Work out the finished part from the listing and answer in its coordinate system (mm). A direction names the side the tool comes from. Give positions to 0.01 mm unless a question says otherwise; leave off trailing zeros. Loops run counter-clockwise (first coordinate to the right, second up) from the corner with the lowest first, then second, coordinate; pieces in that order, holes last. Notation, with made-up numbers: (32.25, 66) -> (87.25, 66) arc R12 cw to (87.25, 80) -> close; hole circle Ø7 at (38.25, 23.5). An arc over 180 degrees is marked (long way). Answer as CSV lines item,"result". Start each with the question number.
1. Determine the mould class of faces 1 (the face through (1, 21, 1.473)), 2 (the face through (28.02, 0.73, 9.95)), 3 (the face through (-33.65, 10.52, 0.75)) for opening direction Z: +Z half, -Z half, draft (parallel to the pull), parting line (faces both ways), or undercut.
2. Find the intervals of material crossed by line 1 along Y through (x, z) = (0.5, 17); line 2 along Z through (x, y) = (30, 1), in increasing order.
3. A tool of negligible diameter and unlimited length cuts with its end or side. For faces 4 (the face through (38.27, 30.52, 0.73)), 5 (the face through (1, 1.473, 21)), from which of +Z, -Z, +X, -X, +Y, -Y can it reach the whole face along a straight path? Write none if from no direction.
4. Flat-ended cylindrical pins translate along their axes: pin 1 Ø5 at (x, y) = (15.5, 13.5) entering from +Z; pin 2 Ø1.5 at (x, z) = (6.5, 9) entering from +Y. Find the tip coordinate at first contact, or state that the pin passes through.
5. Find section A-A, the plane x = 30. Give the vertices of the cut face in (y, z).
6. Find section B-B, the plane y = 18. Give the vertices of the cut face in (x, z), and give its area (3 significant figures).
from build123d import *

# Parameters (mm, degrees)
F1_DEPTH = 50.8
F2_R     = 2.5
F3_DEPTH = 12.7
F4_R     = 2.5
F5_DEPTH = 12.7


with BuildPart() as f1:
    # F0 (on Right) → F1 (new body, symmetric)
    with BuildSketch(Plane.YZ):
        with BuildLine():
            Line((1.4732, 38.1), (0, 38.1))
            Line((0, 38.1), (0, 2.54))
            ThreePointArc((0, 2.54), (0.7439487758, 0.7439487758), (2.54, 0))
            Line((2.54, 0), (38.1, 0))
            Line((38.1, 0), (38.1, 1.4732))
            Line((38.1, 1.4732), (4.0132, 1.4732))
            ThreePointArc((4.0132, 1.4732), (2.2171487758, 2.2171487758), (1.4732, 4.0132))
            Line((1.4732, 4.0132), (1.4732, 38.1))
        make_face()
    extrude(amount=F1_DEPTH, both=True)

    # F2 (on Top) → F3 (cut, symmetric)
    with BuildSketch(Plane.XY):
        with Locations((35.9598398209, 11.4732)):
            Circle(F2_R)
        with Locations((35.9598398209, 31.4732)):
            Circle(F2_R)
        with Locations((-35.9598398209, 31.4732)):
            Circle(F2_R)
        with Locations((-35.9598398209, 11.4732)):
            Circle(F2_R)
    extrude(amount=F3_DEPTH, both=True, mode=Mode.SUBTRACT)

    # F4 (on Front) → F5 (cut, symmetric)
    with BuildSketch(Plane.XZ):
        with Locations((-30, 11.4732)):
            Circle(F4_R)
        with Locations((30, 11.4732)):
            Circle(F4_R)
    extrude(amount=F5_DEPTH, both=True, mode=Mode.SUBTRACT)


solid = f1.part
Resolved:
1,face 1,"+Z half"
1,face 2,"undercut"
1,face 3,"draft"
2,line 1,"y = 0 to 1.47"
2,line 2,"z = 0.52 to 8.97, 13.97 to 38.1"
3,face 4,"+Z, -Z"
3,face 5,"+Z, +X, -X, +Y"
4,pin 1,"stops at z = 1.47"
4,pin 2,"stops at y = 1.47"
5,outline,"(0, 2.54) arc R2.54 ccw to (2.54, 0) -> (38.1, 0) -> (38.1, 1.47) -> (4.01, 1.47) arc R2.54 cw to (1.47, 4.01) -> (1.47, 8.97) -> (0, 8.97) -> close; (0, 13.97) -> (1.47, 13.97) -> (1.47, 38.1) -> (0, 38.1) -> close"
6,outline,"(-50.8, 0) -> (50.8, 0) -> (50.8, 1.47) -> (-50.8, 1.47) -> close"
6,area,"150 mm^2"
